Autodesk Inventor part; units mm, degrees
ref_plane "YZ Plane" through (0, 0, 0) normal (1, 0, 0) x (0, 1, 0)
ref_plane "XZ Plane" through (0, 0, 0) normal (0, 1, 0) x (-1, 0, 0)
ref_plane "XY Plane" through (0, 0, 0) normal (0, 0, 1) x (1, 0, 0)
sketch "Skizze1" plane through (0, 0, 0) normal (0, 0, 1) x (1, 0, 0)
  line L0 (0, 0) -> (0, 10)
  line L1 (0, 10) -> (1.6, 10)
  line L2 (1.6, 10) -> (1.6, 8)
  line L3 (1.6, 8) -> (13.1, 8)
  line L4 (13.1, 8) -> (13.1, 4)
  line L5 (0, 0) -> (12, 0)
  line L6 (13.1, 4) -> (12, 4)
  line L7 (12, 4) -> (12, 0)
  dimension "d0" = 16
  dimension "d1" = 20
  dimension "d2" = 11.5
  dimension "d3" = 1.6
  dimension "d12" = 8
  dimension "d13" = 10.4
revolve "Umdrehung1" add sketch "Skizze1" angle 360 about axis through (0, 0, 0) along (1, 0, 0)
sketch "Skizze2" plane through (0, 0, 0) normal (-1, 0, 0) x (0, 0, 1)
  point P0 (0, 0)
  point P1 (0, 0)
hole "Bohrung1" at (0, 0, 0) direction (1, 0, 0) diameter 4.134 depth 14.2 tip angle 118
feature "Verdickung1" [suppressed]
thicken "Verdickung2" operation add thickness 0.1 both sides no extend neighbours yes toward (0, 0.9870503, -0.1604113) faces at (12.7333, 3.9482, -0.6416)
properties part number "SpringCompensation_Innside_SupportPart" material "PBT-Kunststoff"
Here's how the part is built. I have some questions about the finished solid (model axes, mm). A direction names the side the tool comes from. Round coordinates to 2 decimals unless told otherwise and drop trailing zeros. Order: outer loops, then holes, each group sorted by start corner. A loop starts at its lowest first (then second) coordinate and runs counter-clockwise, first axis right, second up. Notation, with made-up numbers: M 70,75.5 L 110,75.5 A24 ccw 110,112.5 Z; hole C 84.5,82.5 d3. An arc over 180 degrees is marked long. Answer in a Markdown table with one row per item.
Item 1: If I drill on L1, parallel to Z at x = 5.5, y = 0; L2, parallel to Z at x = 12.3, y = 0; L3, parallel to X at y = -0.5, z = 3.75, over which ranges is the centre line in solid material (lowest first)? Write a range as from..to.
A:
| item | result |
|---|---|
| L1 | z = -8..-2.07, 2.07..8 |
| L2 | z = -8..-4.1, 4.1..8 |
| L3 | x = 0..12 |
Item 2: Thinking about a two-plate mould opening in Y: for faces 3 (the face through (7.43, -1.73, -7.81)), 4 (the face through (12, -2, 1)), 5 (the face through (1.6, 0, 8.2)), which applies, +Y half, -Y half, draft (parallel to the pull), parting line (faces both ways), or undercut?
A:
| item | result |
|---|---|
| face 3 | parting line |
| face 4 | undercut |
| face 5 | draft |
Item 3: Imagine slicing it at C-C, the plane x = 8. Write out the boundary of the cut face in (y, z).
A:
| item | result |
|---|---|
| outline | C 0,0 d16; hole C 0,0 d4.13 |
Item 4: I'm going to push flat-ended pins straight in: pin 1 (5 mm diameter, centred on x = 10, z = -3, fed in from +Y); pin 2 (6 mm diameter, centred on x = 10, y = 8, fed in from -Z) (3 decimals); pin 3 (1.5 mm diameter, centred on x = 3, y = -1, fed in from +Z); pin 4 (3.5 mm diameter, centred on y = 0, z = 0, fed in from -X). Where does each tip first touch, or does it pass through?
A:
| item | result |
|---|---|
| pin 1 | stops at y = 7.98 |
| pin 2 | stops at z = -6.245 |
| pin 3 | stops at z = 8 |
| pin 4 | passes through |
Item 5: For faces 1 (the face through (13.1, -4, 2)), 2 (the face through (12.542, -0.534, -4.065)), which set-ups out of +Z, -Z, +X, -X, +Y, -Y let a thin tool reach every point of the face, with its end or its side?
A:
| item | result |
|---|---|
| face 1 | +Z, -Z, +X, +Y, -Y |
| face 2 | +X |
Item 6: Imagine slicing it at D-D, the plane y = 6.25. Write out the boundary of the cut face in (x, z).
A:
| item | result |
|---|---|
| outline | M 0,-7.81 L 1.6,-7.81 L 1.6,-4.99 L 13.1,-4.99 L 13.1,4.99 L 1.6,4.99 L 1.6,7.81 L 0,7.81 Z |
Item 7: Imagine slicing it at A-A, the plane y = 0. Write out the boundary of the cut face in (x, z).
A:
| item | result |
|---|---|
| outline | M 0,-10 L 1.6,-10 L 1.6,-8 L 13.1,-8 L 13.1,-4.1 L 12,-4.1 L 12,-2.07 L 0,-2.07 Z; M 0,2.07 L 12,2.07 L 12,4.1 L 13.1,4.1 L 13.1,8 L 1.6,8 L 1.6,10 L 0,10 Z |
